Source: CAD feature listing. Evaluate the final solid. Frame: model axes, mm. A direction names the side the tool comes from. Give positions to 0.01 mm unless a question says otherwise; leave off trailing zeros. Answer in a Markdown table with one row per item. Add a question column.
(1) Pin query (flat end, axial travel): P1, Ø6, axis at x = 25.5, z = 51, coming from the +Y side; P2, Ø10, axis at x = 29.5, z = 10.5, coming from the -Y side; P3, Ø19.5, axis at x = -6, y = -4.5, coming from the +Z side; P4, Ø4, axis at x = -25.5, y = 20.5, coming from the -Z side. Return the tip coordinate at first contact, or that it passes through.
(2) Material intervals for line 1 along Z through (x, y) = (-7.5, 29); line 2 along Y through (x, z) = (0, 85.5); line 3 along Z through (x, y) = (2, -29), sorted ascending.
(3) Mould query, pull axis Y, two halves, no side actions, for faces 4 (the face through (0, 1, 2.54)), 5 (the face through (0, 1, 0)), 6 (the face through (-21.53, 19.74, 82.46)). Classes: pulls with the +Y half, pulls with the -Y half, needs draft (parallel to the pull), parting line crosses it, or undercut.
(4) Set-up query: faces 1 (the face through (-3.472, 26.443, 81.173)), 2 (the face through (24, -12, 73.66)), 3 (the face through (13, -24, 88.9)). Return all of +Z, -Z, +X, -X, +Y, -Y with unobstructed straight access to the full face (end or side cutting, diameter ignored); none if empty.
from build123d import *

# Parameters (mm, degrees)
F4_R     = 29.21
F5_DEPTH = 12.7
F6_T     = -2.54


with BuildPart() as f3:
    # F0 (on Top) → F3 section 0
    with BuildSketch(Plane.XY):
        Polygon((18.4117928475, 44.45), (-18.4117928475, 44.45), (-44.45, 18.4117928475), (-44.45, -18.4117928475), (-18.4117928475, -44.45), (18.4117928475, -44.45), (44.45, -18.4117928475), (44.45, 18.4117928475), align=None)
    # F2 (on offset) → F3 section 1
    with BuildSketch(Plane.XY.offset(76.2)):
        Polygon((32.8531561761, -13.6082228549), (32.8531561761, 13.6082228549), (13.6082228549, 32.8531561761), (-13.6082228549, 32.8531561761), (-32.8531561761, 13.6082228549), (-32.8531561761, -13.6082228549), (-13.6082228549, -32.8531561761), (13.6082228549, -32.8531561761), align=None)
    loft()

    # F4 (on face) → F5 (join)
    with BuildSketch(Plane.XY.offset(76.2)):
        Circle(F4_R)
    extrude(amount=F5_DEPTH)

    # F6
    f6_openings = [f3.faces().sort_by_distance(p)[0] for p in [
        (0, 0, 88.9),
    ]]
    offset(amount=F6_T, openings=f6_openings, kind=Kind.INTERSECTION)


solid = f3.part
Values follow:
| question | item | result |
|---|---|---|
| 1 | P1 | stops at y = 29.45 |
| 1 | P2 | stops at y = -36.22 |
| 1 | P3 | stops at z = 2.54 |
| 1 | P4 | stops at z = 0 |
| 2 | line 1 | z = 0 to 2.54, 73.66 to 76.2 |
| 2 | line 2 | y = -29.21 to -26.67, 26.67 to 29.21 |
| 2 | line 3 | z = 0 to 2.54, 73.66 to 88.9 |
| 3 | face 4 | undercut |
| 3 | face 5 | needs draft |
| 3 | face 6 | parting line crosses it |
| 4 | face 1 | +Z |
| 4 | face 2 | none |
| 4 | face 3 | +Z, +X, -X, +Y, -Y |
